Could you check a few things on this model? Use its own coordinates, in mm. A direction names the side the tool comes from. Coordinates: 2 decimals unless noted, no trailing zeros. Loops run counter-clockwise (first coordinate to the right, second up) from the corner with the lowest first, then second, coordinate; pieces in that order, holes last.
1) Will these pins go through, and if not, where does the flat tip stop? P1, Ø10, axis at y = -13.5, z = 2.5, coming from the -X side; P2, Ø4, axis at x = -7, z = -14, coming from the +Y side; P3, Ø8, axis at x = 15.5, y = 14, coming from the +Z side.
2) Imagine slicing it at B-B on z = -26. Please give me the cut outline in (x, y), plus the area to 3 significant figures.
3) Thinking about a two-plate mould opening in Z: for faces 1 (the face through (1.979, -15.071, -19.078)), 2 (the face through (0.788, 3.547, 47.165)), 3 (the face through (19.75, 15.15, -35.66)), which applies, released by +Z, released by -Z, zero draft, split by the parting line, or undercut?
4) Imagine slicing it at A-A on z = 41.5. Please give me the cut outline in (x, y).
5) If I drill on line 1 along Z through (x, y) = (-19.5, -6); line 2 along Z through (x, y) = (17, 9); line 3 along Z through (x, y) = (-8.5, -5), over which ranges is the centre line in solid material (lowest first)?
6) For faces 4 (the face through (-19.975, -6.29, 25.118)), 5 (the face through (1, 0.7, -38.1)), 6 (the face through (1.965, -14.97, 15.673)), which set-ups out of +Z, -Z, +X, -X, +Y, -Y let a thin tool reach every point of the face, with its end or its side?
```python
from build123d import *


with BuildPart() as f1:
    # F0 (on Front) → F1 (revolve)
    with BuildSketch(Plane.XZ):
        Polygon((0, 34.8173603415), (0, 49.7604347765), (-20.9203045815, 34.8173603415), align=None)
        Polygon((0, 34.8173603415), (-20.9203045815, 34.8173603415), (-20.9630057216, 15.6858414412), (-14.7989457213, 15.6720833914), (0, 15.6390524618), align=None)
        Polygon((0, -38.0559399025), (0, 15.6390524618), (-14.7989457213, 15.6720833914), (-14.8749074655, -18.3612829992), (-20.0824216008, -29.8110116273), (-25.0723995268, -30.3980689496), (-24.7788708657, -38.9103852212), align=None)
    revolve(axis=Axis((0, 0, -11.2084437204), (0, 0, 1)))


solid = f1.part
```
Filled in:
1. P1: stops at x = -12.15
1. P2: stops at y = 14
1. P3: stops at z = 37.7
2. outline: circle Ø36.7 at (0, 0)
2. area: 1,060 mm2
3. face 1: undercut
3. face 2: released by +Z
3. face 3: released by -Z
4. outline: circle Ø23.13 at (0, 0)
5. line 1: z = -38.76 to -29.85, 15.68 to 35.19
5. line 2: z = -38.72 to -27.95, 15.68 to 36.02
5. line 3: z = -38.4 to 42.72
6. face 4: +Z
6. face 5: -Z
6. face 6: none
